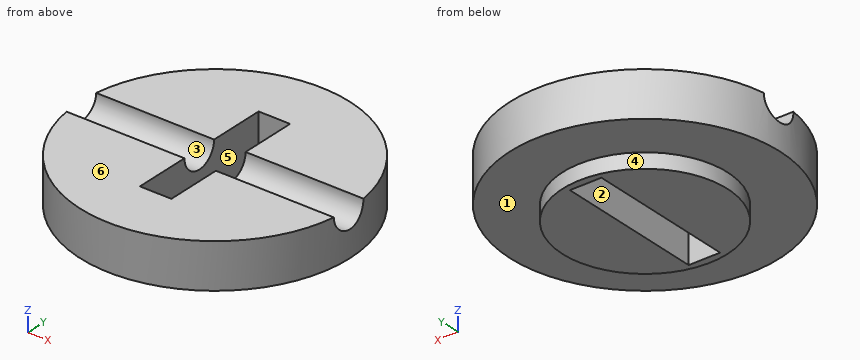
from build123d import *

# Parameters (mm, degrees)
F0_R     = 9
F1_DEPTH = 3
F2_R     = 5.5
F3_DEPTH = 1
F4_R     = 1.25
F5_DEPTH = 9
F6_W     = 2.1
F6_H     = 3.75
F6_H_2   = 2.5
F7_DEPTH = 4.001


# Not quite as in the source:
# - a feature names something its author has since deleted; it is built from what else it names


with BuildPart() as f1:
    # F0 (on Top) → F1 (new body)
    with BuildSketch(Plane.XY):
        Circle(F0_R)
    extrude(amount=-F1_DEPTH)

    # F2 (on face) → F3 (join)
    with BuildSketch(Plane(origin=(0, 0, -3), x_dir=(1, 0, 0), z_dir=(0, 0, -1))):
        Circle(F2_R)
    extrude(amount=F3_DEPTH)

    # F4 (on Right) → F5 (cut, symmetric)
    with BuildSketch(Plane.YZ):
        Circle(F4_R)
    extrude(amount=F5_DEPTH, both=True, mode=Mode.SUBTRACT)

    # F6 (on face) → F7 (cut, through all)
    with BuildSketch(Plane.XY):
        with Locations((0, -3.125)):
            Rectangle(F6_W, F6_H)
        Rectangle(F6_W, F6_H_2)
        with Locations((0, 3.125)):
            Rectangle(F6_W, F6_H)
    extrude(amount=-F7_DEPTH, mode=Mode.SUBTRACT)


solid = f1.part
The listing builds one solid part. Answer for the finished solid, in the listing's coordinates (mm). Face numbers are marked on the shaded views. A direction names the side the tool comes from. Round coordinates to 2 decimals unless told otherwise and drop trailing zeros. Order: outer loops, then holes, each group sorted by start corner. A loop starts at its lowest first (then second) coordinate and runs counter-clockwise, first axis right, second up. Notation, with made-up numbers: M 82.5,-22.75 L 97.5,-22.75 A17 cw 97.5,-9.75 Z; hole C -6,35.5 d9. An arc over 180 degrees is marked long. Answer in a Markdown table with one row per item. Add a question column.
1) Flat-ended cylindrical pins translate along their axes: pin 1 Ø1.2 at (y, z) = (2.5, -2) entering from +X; pin 2 Ø2 at (x, y) = (7, 0.5) entering from -Z; pin 3 Ø1 at (x, y) = (3, 0) entering from +Z. Find the tip coordinate at first contact, or state that the pin passes through.
2) The part is cut by section B-B on z = -2. Determine the outline of the cut face in (x, y), plus the area to 3 significant figures.
3) Determine the mould class of the marked faces 4, 5 and 6 for opening direction X: pulls with the +X half, pulls with the -X half, needs draft (parallel to the pull), parting line crosses it, or undercut.
4) Which of the six approach directions +Z, -Z, +X, -X, +Y, -Y give full straight-line access (tool end or side, diameter ignored) to the marked faces 1, 2 and 3?
5) The part is cut by section C-C on x = 0. Determine the outline of the cut face in (y, z), plus the area to 3 significant figures.
6) The part is cut by section D-D on x = 4. Determine the outline of the cut face in (y, z).
7) The part is cut by section A-A on y = 0. Determine the outline of the cut face in (x, z).
8) Consider line 1 along Y through (x, z) = (0, -3.25); line 2 along X through (y, z) = (4, -1.45); line 3 along X through (y, z) = (-4.25, -1.35). Determine where each line is inside the solid, lowest interval first. Write a range as from..to.
Findings below:
| question | item | result |
|---|---|---|
| 1 | pin 1 | stops at x = 8.8 |
| 1 | pin 2 | stops at z = -3 |
| 1 | pin 3 | stops at z = -1.15 |
| 2 | outline | C 0,0 d18; hole M -1.05,-5 L 1.05,-5 L 1.05,5 L -1.05,5 Z |
| 2 | area | 233 mm² |
| 3 | face 4 | parting line crosses it |
| 3 | face 5 | undercut |
| 3 | face 6 | needs draft |
| 4 | face 1 | -Z |
| 4 | face 2 | +Z, -Z |
| 4 | face 3 | +Z, +X, -X |
| 5 | outline | M -9,-3 L -5.5,-3 L -5.5,-4 L -5,-4 L -5,0 L -9,0 Z; M 5,-4 L 5.5,-4 L 5.5,-3 L 9,-3 L 9,0 L 5,0 Z |
| 5 | area | 25.0 mm² |
| 6 | outline | M -8.06,-3 L -3.77,-3 L -3.77,-4 L 3.77,-4 L 3.77,-3 L 8.06,-3 L 8.06,0 L 1.25,0 A1.25 cw -1.25,0 L -8.06,0 Z |
| 7 | outline | M -9,-3 L -5.5,-3 L -5.5,-4 L -1.05,-4 L -1.05,-1.25 L -9,-1.25 Z; M 1.05,-4 L 5.5,-4 L 5.5,-3 L 9,-3 L 9,-1.25 L 1.05,-1.25 Z |
| 8 | line 1 | y = -5.5..-5, 5..5.5 |
| 8 | line 2 | x = -8.06..-1.05, 1.05..8.06 |
| 8 | line 3 | x = -7.93..-1.05, 1.05..7.93 |
